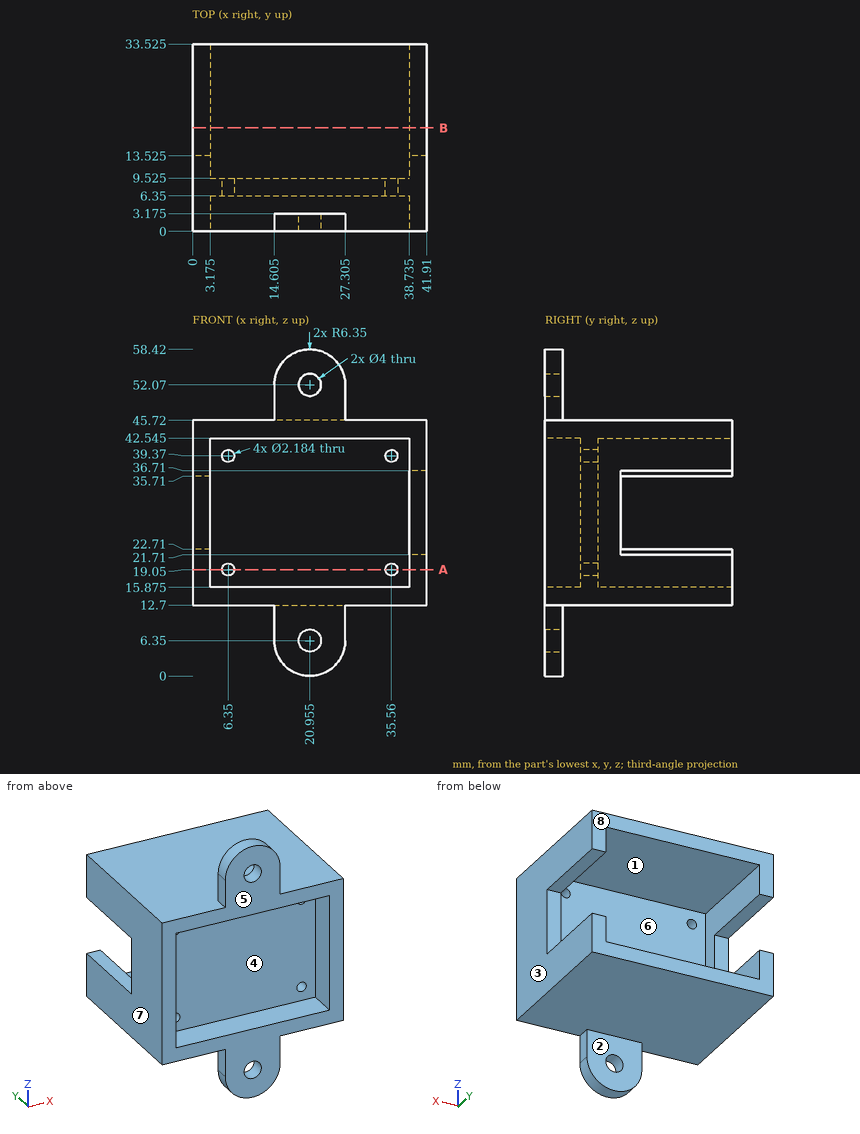
Check sheet for the drawn part. Datum: minimum x, y, z corner. Units: mm. A direction names the side the tool comes from. Round coordinates to 2 decimals unless told otherwise and drop trailing zeros. Order: outer loops, then holes, each group sorted by start corner. A loop starts at its lowest first (then second) coordinate and runs counter-clockwise, first axis right, second up. Notation, with made-up numbers: (64.25, -39) -> (91.25, -39) arc R8 ccw to (91.25, -29) -> close; hole circle Ø2 at (60, 34). An arc over 180 degrees is marked (long way). Put each result on its own line as item: value. Start each with the question number.
(1) Material ranges on line 1 along X through (y, z) = (8.75, 19.05); line 2 along X through (y, z) = (1.3, 52.07) (1 decimal); line 3 along Z through (x, y) = (37, 6) (1 decimal), recorded low to high.
(2) Depth check by flat-ended pin: pin 1 Ø1 at (y, z) = (2, 10) entering from -X (3 decimals); pin 2 Ø10 at (x, y) = (23.5, 12) entering from +Z; pin 3 Ø1.6 at (x, z) = (2.5, 28) entering from +Y (3 decimals); pin 4 Ø4 at (y, z) = (24.5, 33) entering from +X. Enter the tip coordinate at first touch or a pass-through.
(3) Draft check along X on the marked faces 6, 7 and 8. Enter one of: +X half, -X half, draft (parallel to the pull), parting line (faces both ways), or undercut.
(4) Section check B-B (y = 18.5). Enter the section's corners in (x, z) (1 decimal).
(5) Tool access check on the marked faces 1, 2, 3, 4 and 5. Record the directions out of +Z, -Z, +X, -X, +Y, -Y that give a thin tool (end or side, any length) a straight path to the whole face; none if there is none.
(6) Section check A-A (z = 19.05). State how many separate pieces and enclosed holes the cut face has, then the cut area to 3 significant figures.
Completed:
1. line 1: x = 0 to 5.26, 7.44 to 34.47, 36.65 to 41.91
1. line 2: x = 14.6 to 19, 23 to 27.3
1. line 3: z = 12.7 to 15.9, 42.5 to 45.7
2. pin 1: stops at x = 14.605
2. pin 2: stops at z = 45.72
2. pin 3: stops at y = 13.525
2. pin 4: passes through
3. face 6: undercut
3. face 7: -X half
3. face 8: draft
4. outline: (0, 12.7) -> (41.9, 12.7) -> (41.9, 21.7) -> (38.7, 21.7) -> (38.7, 15.9) -> (3.2, 15.9) -> (3.2, 22.7) -> (0, 22.7) -> close; (0, 35.7) -> (3.2, 35.7) -> (3.2, 42.5) -> (38.7, 42.5) -> (38.7, 36.7) -> (41.9, 36.7) -> (41.9, 45.7) -> (0, 45.7) -> close
5. face 1: +Y
5. face 2: -Z, +X, -X, +Y
5. face 3: +Z, -Z, +X, +Y, -Y
5. face 4: -Y
5. face 5: +Z, -Z, +X, -X, -Y
6. separate pieces: 3
6. enclosed holes: 0
6. area: 312 mm2
